Verification items for this drawing (mm, ordinates from the low corner). A direction names the side the tool comes from. Give positions to 0.01 mm unless a question says otherwise; leave off trailing zeros. Write each loop counter-clockwise with the first axis right and the second up, starting at its lowest first coordinate (ties: lowest second). Pieces come first, ordered by that corner, then holes. Notation, with made-up numbers: (73, -3.75) -> (93, -3.75) arc R10 cw to (93, 5.25) -> close; hole circle Ø3 at (25.25, -27.5). An arc over 180 degrees is marked (long way). One line per item, written item: value.
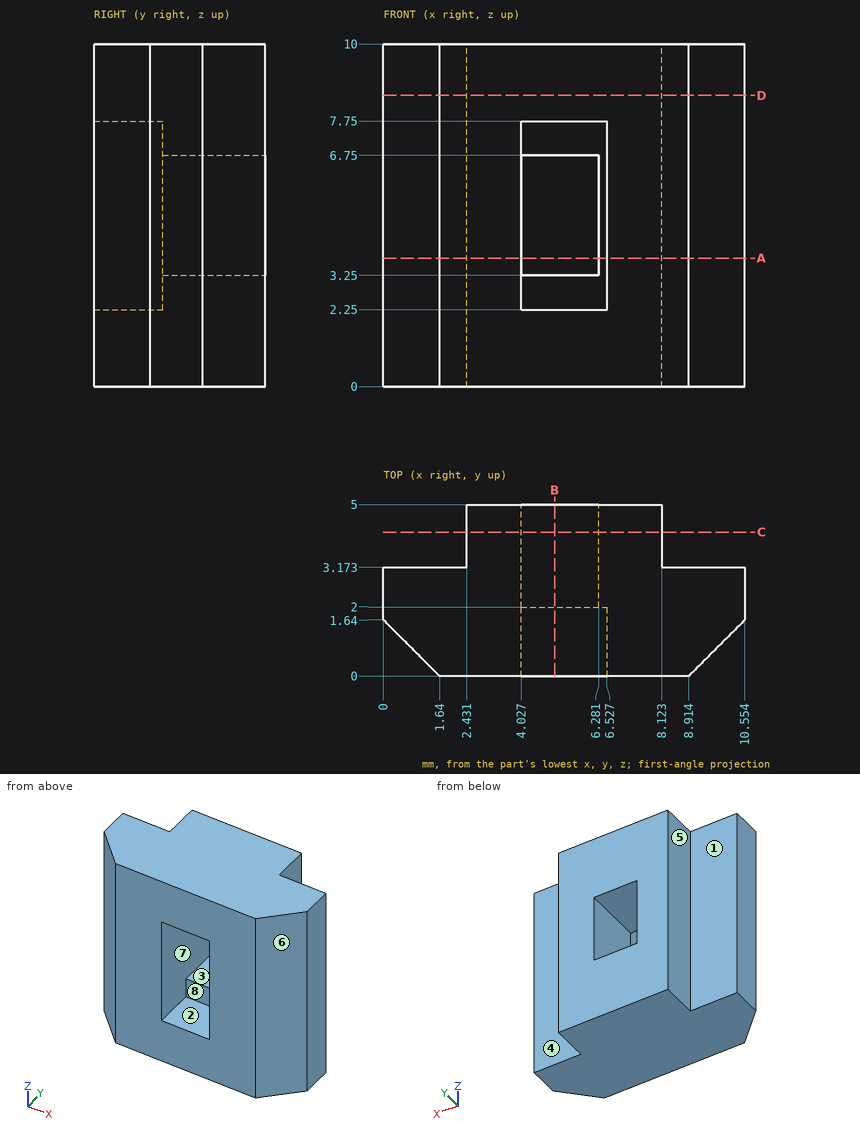
1) Depth check by flat-ended pin: pin 1 Ø2 at (y, z) = (4.5, 3) entering from -X; pin 2 Ø3 at (x, z) = (5, 6) entering from -Y. Enter the tip coordinate at first touch or a pass-through.
Verdict:
pin 1: x = 2.43
pin 2: y = 0
2) Tool access check on the marked faces 1, 2, 3 and 4. Record the directions out of +Z, -Z, +X, -X, +Y, -Y that give a thin tool (end or side, any length) a straight path to the whole face; none if there is none.
Verdict:
face 1: +Z, -Z, -X, +Y
face 2: -Y
face 3: +Y, -Y
face 4: +Z, -Z, +X, +Y
3) Sectioned sample at B-B on x = 5. Record the cut outline in (y, z).
Verdict:
outline: (0, 0) -> (5, 0) -> (5, 3.25) -> (2, 3.25) -> (2, 2.25) -> (0, 2.25) -> close; (0, 7.75) -> (2, 7.75) -> (2, 6.75) -> (5, 6.75) -> (5, 10) -> (0, 10) -> close
4) Sectioned sample at C-C on y = 4.2. Record the cut outline in (x, z).
Verdict:
outline: (2.43, 0) -> (8.12, 0) -> (8.12, 10) -> (2.43, 10) -> close; hole (4.03, 3.25) -> (6.28, 3.25) -> (6.28, 6.75) -> (4.03, 6.75) -> close
5) Mould release check, pull along X, two halves, no side actions. Record for the marked faces 5, 6, 7 and 8: released by +X, released by -X, zero draft, split by the parting line, or undercut.
Verdict:
face 5: released by -X
face 6: released by +X
face 7: undercut
face 8: undercut
6) Sectioned sample at D-D on z = 8.5. Record the cut outline in (x, y), plus the area to 3 significant figures.
Verdict:
outline: (0, 1.64) -> (1.64, 0) -> (8.91, 0) -> (10.55, 1.64) -> (10.55, 3.17) -> (8.12, 3.17) -> (8.12, 5) -> (2.43, 5) -> (2.43, 3.17) -> (0, 3.17) -> close
area: 41.2 mm^2
7) Sectioned sample at A-A on z = 3.75. Record the cut outline in (x, y).
Verdict:
outline: (0, 1.64) -> (1.64, 0) -> (4.03, 0) -> (4.03, 5) -> (2.43, 5) -> (2.43, 3.17) -> (0, 3.17) -> close; (6.28, 2) -> (6.53, 2) -> (6.53, 0) -> (8.91, 0) -> (10.55, 1.64) -> (10.55, 3.17) -> (8.12, 3.17) -> (8.12, 5) -> (6.28, 5) -> close
8) Scan lines: probe 1 along Z at (x, y) = (5, 0.8); probe 2 along X at (y, z) = (2.95, 6.5); probe 3 along Z at (x, y) = (6.25, 2.7). Record each from-to range of solid material in increasing order.
Verdict:
probe 1: 0 to 2.25, 7.75 to 10
probe 2: 0 to 4.03, 6.28 to 10.55
probe 3: 0 to 3.25, 6.75 to 10
